from build123d import *

# Parameters (mm, degrees)
SKETCH1_W           = 15
SKETCH1_H           = 15
BOSS_EXTRUDE1_DEPTH = 5
SKETCH5_R           = 4
BOSS_EXTRUDE3_DEPTH = 10
BOSS_EXTRUDE4_DEPTH = 5


with BuildPart() as part:
    # Sketch1 → Boss-Extrude1 (new body)
    with BuildSketch(Plane(origin=(0, 0, 0), x_dir=(1, 0, 0), z_dir=(0, 1, 0))):
        Rectangle(SKETCH1_W, SKETCH1_H)
    extrude(amount=BOSS_EXTRUDE1_DEPTH)

    # Sketch5 → Boss-Extrude3 (add)
    with BuildSketch(Plane.XZ):
        with Locations(Location((0, 0, 0), (0, 0, 270))):
            Circle(SKETCH5_R)
    extrude(amount=BOSS_EXTRUDE3_DEPTH)

    # Sketch6 → Boss-Extrude4 (add)
    with BuildSketch(Plane(origin=(0, 5, 0), x_dir=(1, 0, 0), z_dir=(0, 1, 0))):
        Polygon((-2.542898848, -3.5), (-1.571597918, -0.510643118), (-4.114496766, 1.336881039), (-0.97130093, 1.336881039), (0, 4.326237921), (0.97130093, 1.336881039), (4.114496766, 1.336881039), (1.571597918, -0.510643118), (2.542898848, -3.5), (0, -1.652475842), align=None)
    extrude(amount=BOSS_EXTRUDE4_DEPTH)


solid = part.part
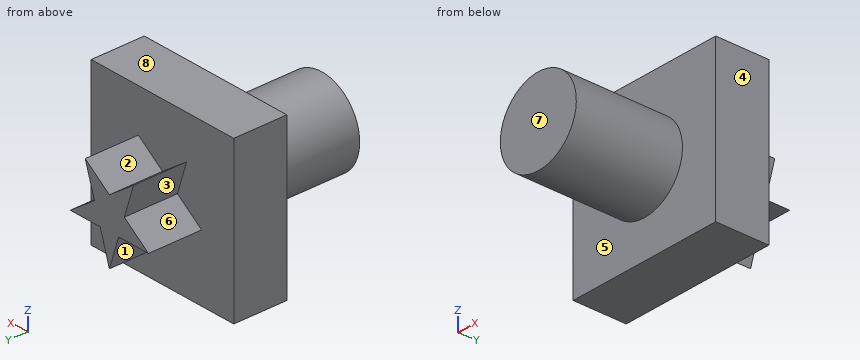
The model under review builds one solid part; all positions refer to its coordinate system, in mm. Face numbers are marked on the shaded views. A direction names the side the tool comes from. Round coordinates to 2 decimals unless told otherwise and drop trailing zeros. Order: outer loops, then holes, each group sorted by start corner. A loop starts at its lowest first (then second) coordinate and runs counter-clockwise, first axis right, second up. Notation, with made-up numbers: (0, -20.75) -> (13, -20.75) arc R11 ccw to (13, -14.75) -> close; hole circle Ø8 at (3, -33.5). An arc over 180 degrees is marked (long way). Return JSON: item names as keys, results as strings.
1. For the marked faces 1, 2, 3, 4 and 5, list the 3-axis set-ups (+Z, -Z, +X, -X, +Y, -Y) from which the entire face can be reached by the end or side of a thin tool; tool diameter is ignored.
Answer block:
{"face 1": "-Z, -X, +Y", "face 2": "+Z, +Y", "face 3": "-X, +Y", "face 4": "+Z, -Z, +X, +Y, -Y", "face 5": "-Y"}
2. For L1, parallel to Y at x = 4.75, z = -2.5; L2, parallel to Y at x = -1.75, z = 3.5; L3, parallel to X at y = -5.5, z = -1.75, list the stretches that pass through material, from the lowest coordinate up. Write a range as [from, to].
Answer block:
{"L1": "y = [0, 5]", "L2": "y = [-10, 5]", "L3": "x = [-3.6, 3.6]"}
3. Take a section at D-D (z = 0). Write out the cut boundary in (x, y).
Answer block:
{"outline": "(-7.5, 0) -> (-4, 0) -> (-4, -10) -> (4, -10) -> (4, 0) -> (7.5, 0) -> (7.5, 5) -> (2.27, 5) -> (2.27, 10) -> (-2.27, 10) -> (-2.27, 5) -> (-7.5, 5) -> close"}
4. The part is to be moulded in two halves that separate along Z. For the marked faces 6, 7 and 8, say which applies: +Z half, -Z half, draft (parallel to the pull), parting line (faces both ways), or undercut.
Answer block:
{"face 6": "undercut", "face 7": "draft", "face 8": "+Z half"}
5. Take a section at A-A (z = -3.25). Write out the cut boundary in (x, y).
Answer block:
{"outline": "(-7.5, 0) -> (-2.33, 0) -> (-2.33, -10) -> (2.33, -10) -> (2.33, 0) -> (7.5, 0) -> (7.5, 5) -> (0.35, 5) -> (0.35, 10) -> (-0.35, 10) -> (-0.35, 5) -> (-7.5, 5) -> close"}
6. Take a section at C-C (y = -2). Write out the cut boundary in (x, z).
Answer block:
{"outline": "circle Ø8 at (0, 0)"}
7. Insertion check: P1, Ø4, axis at x = -0.5, y = -5, coming from the +Z side; P2, Ø0.9, axis at x = 2, y = 8.5, coming from the -Z side; P3, Ø3, axis at x = -1, y = 7.5, coming from the +Z side. Each pin has a flat end and moves straight along its axis. Give the tip position at first contact, or say it passes through.
Answer block:
{"P1": "stops at z = 4", "P2": "stops at z = -1.34", "P3": "stops at z = 3.47"}
8. Take a section at B-B (x = 2). Write out the cut boundary in (y, z).
Answer block:
{"outline": "(-10, -3.46) -> (0, -3.46) -> (0, -7.5) -> (5, -7.5) -> (5, -1.34) -> (10, -1.34) -> (10, 0.2) -> (5, 0.2) -> (5, 1.83) -> (10, 1.83) -> (10, 3.11) -> (5, 3.11) -> (5, 7.5) -> (0, 7.5) -> (0, 3.46) -> (-10, 3.46) -> close"}
